Design review of the part built by this model. Coordinates are the model's own, in mm. A direction names the side the tool comes from. Give positions to 0.01 mm unless a question says otherwise; leave off trailing zeros. Write each loop counter-clockwise with the first axis right and the second up, starting at its lowest first coordinate (ties: lowest second). Pieces come first, ordered by that corner, then holes. Notation, with made-up numbers: (71, 3.25) -> (121, 3.25) arc R11 cw to (121, 19.25) -> close; hole circle Ø5 at (77.25, 57.5). An arc over 180 degrees is marked (long way). Write each question's results on one line, items separated by ' | '. Start each with the question number.
(1) Mouldability with a two-part tool opening along X and no side actions: class faces 1 (the face through (62.402, 13, 9)), 2 (the face through (-15.24, 1.65, 15.07)), 3 (the face through (23, 15, 20)) as released by +X, released by -X, zero draft, split by the parting line, or undercut.
(2) Take a section at C-C (z = 7.25). Count the separate pieces of the cut face and the enclosed holes in it, plus the area to 3 significant figures.
(3) Take a section at A-A (z = 12.75). State the section outline as (x, y) points.
(4) Take a section at B-B (y = 22). State the section outline as (x, z) points, plus the area to 3 significant figures.
(5) Clearance check with flat-ended pins moving along their axes: pin 1 (1.2 mm diameter, centred on y = 1.5, z = 4.5, fed in from -X); pin 2 (1.2 mm diameter, centred on x = 42, z = 6.5, fed in from -Y); pin 3 (1.2 mm diameter, centred on x = 12.5, y = 3, fed in from -Z). State where each tip first meets the part, or that it passes through.
(6) For faces 4 (the face through (57.165, 16.022, 5.07)), 5 (the face through (62.4, 31.32, 8.38)), 6 (the face through (16, 2, 10)), list the 3-axis set-ups (+Z, -Z, +X, -X, +Y, -Y) from which the entire face can be reached by the end or side of a thin tool; tool diameter is ignored.
(7) To check wall thickness, follow probe 1 along Y at (x, z) = (58.9, 5.25); probe 2 along Y at (x, z) = (42.4, 2.25); probe 3 along X at (y, z) = (8, 4.75). State the ranges of each line that lie inside material, in increasing order.
Autodesk Inventor part; units mm, degrees
ref_plane "YZ Plane" through (0, 0, 0) normal (1, 0, 0) x (0, 1, 0)
ref_plane "XZ Plane" through (0, 0, 0) normal (0, 1, 0) x (-1, 0, 0)
ref_plane "XY Plane" through (0, 0, 0) normal (0, 0, 1) x (1, 0, 0)
ref_plane "Arbeitsebene1" through (0, 0, 0) normal (0, 0, 1) x (1, 0, 0)
sketch "Skizze1" plane through (0, 0, 0) normal (0, 0, 1) x (1, 0, 0)
  line L0 (37.9, 26.5) -> (37.9, 13.35)
  line L1 (37.9, 13.35) -> (53.9, 13.35)
  line L2 (53.9, 13.35) -> (53.9, 13.85)
  line L3 (53.9, 13.85) -> (63.9, 13.85)
  line L4 (63.9, 13.85) -> (63.9, 27.75)
  arc A0 (63.9, 27.75) -> (58.9, 32.75) centre (58.9, 27.75) ccw
  line L5 (58.9, 32.75) -> (-58.9, 32.75)
  arc A1 (-58.9, 32.75) -> (-63.9, 27.75) centre (-58.9, 27.75) ccw
  line L6 (-63.9, 27.75) -> (-63.9, 19.25)
  line L7 (-63.9, 19.25) -> (-58.9, 19.25)
  line L8 (-58.9, 19.25) -> (-58.9, 19.75)
  line L9 (-58.9, 19.75) -> (-38.9, 19.75)
  line L10 (-38.9, 19.75) -> (-38.9, 13.85)
  line L11 (-38.9, 13.85) -> (-28.9, 13.85)
  line L12 (-28.9, 13.85) -> (-28.9, 13.35)
  line L13 (-28.9, 13.35) -> (-8.6, 13.35)
  line L14 (-8.6, 13.35) -> (-8.6, 26.5)
  line L15 (-8.6, 26.5) -> (37.9, 26.5)
  circle A2 centre (58.6204, 27.75) radius 1.4
  circle A3 centre (-59.1796, 27.75) radius 1.4
  circle A4 centre (-13.6, 16.25) radius 1.4
  circle A5 centre (-33.6, 16.25) radius 1.4
  circle A6 centre (58.9, 16.25) radius 1.4
  circle A7 centre (42.4, 16.25) radius 1.4
  line L16 (-8.6, -11.9682) -> (-10.6, -13.9682)
  line L17 (-8.6, -11.9682) -> (-8.6, 5.15)
  line L18 (-8.6, 5.15) -> (-28.9, 5.15)
  line L19 (-28.9, 5.15) -> (-28.9, 4.65)
  line L20 (-28.9, 4.65) -> (-38.9, 4.65)
  line L21 (-38.9, 4.65) -> (-38.9, -1.25)
  line L22 (-38.9, -1.25) -> (-58.9, -1.25)
  line L23 (-58.9, -1.25) -> (-58.9, -0.75)
  line L24 (-58.9, -0.75) -> (-63.9, -0.75)
  line L25 (-63.9, -0.75) -> (-63.9, -16.5797)
  arc A8 (-49.9, -11.2196) -> (-63.9, -16.5797) centre (-50.2702, -31.2162) ccw
  line L26 (-49.9, -11.2196) -> (-49.9, -13.9682)
  line L27 (-49.9, -13.9682) -> (-10.6, -13.9682)
  circle A9 centre (-13.3796, -11.2637) radius 1.4
  circle A10 centre (-33.6, 2.25) radius 1.4
  circle A11 centre (-13.6, 2.25) radius 1.4
  circle A12 centre (58.6204, -47.75) radius 1.4
  circle A13 centre (58.9, 2.25) radius 1.4
  circle A14 centre (42.4, 2.25) radius 1.4
  circle A15 centre (42.4, -11.2637) radius 1.4
  circle A16 centre (42.4, -31.25) radius 1.4
  line L28 (63.9, 4.65) -> (53.9, 4.65)
  line L29 (53.9, 4.65) -> (53.9, 5.15)
  line L30 (53.9, 5.15) -> (37.9, 5.15)
  line L31 (37.9, 5.15) -> (37.9, -41.35)
  line L32 (37.9, -41.35) -> (-33.0276, -41.35)
  arc A17 (-59.1255, -49.149) -> (-33.0276, -41.35) centre (-50.2702, -31.2162) ccw
  arc A18 (-60.3777, -48.4742) -> (-59.1255, -49.149) centre (-59.1796, -47.75) ccw
  arc A19 (-63.9, -45.8527) -> (-60.3777, -48.4742) centre (-50.2702, -31.2162) ccw
  line L33 (-63.9, -45.8527) -> (-63.9, -47.75)
  arc A20 (-63.9, -47.75) -> (-58.9, -52.75) centre (-58.9, -47.75) ccw
  line L34 (-58.9, -52.75) -> (58.9, -52.75)
  arc A21 (58.9, -52.75) -> (63.9, -47.75) centre (58.9, -47.75) ccw
  line L35 (63.9, -47.75) -> (63.9, 4.65)
  line L36 (-16.1, 32.75) -> (63.9, 32.75)
  line L37 (63.9, 32.75) -> (63.9, 0.75)
  line L38 (63.9, 0.75) -> (-16.1, 0.75)
  line L39 (-16.1, 0.75) -> (-16.1, 32.75)
  point P0 (0, 0)
  dimension "d0" = 80
  dimension "d1" = 0
  dimension "d2" = 32
extrude "Extrusion1" add sketch "Skizze1" along normal blind 20 contours L15 L14 L13 L39 L5 A0 L4 L3 L2 L1 L0 | L0 L1 L2 L3 L37 L28 L29 L30 L31 L38 L17 L18 L39 L13 L14 L15 | L18 L17 L38 L39 | L35 L38 L31 L30 L29 L28 | A2 | A4 | A6 | A7 | A11 | A13 | A14
fillet "Rundung1" radius 3 7 edges at (62.4355, 31.2855, 20) (63.9, 20.8, 20) (21.4, 32.75, 20) (-16.1, 16.75, 20) (-16.1, 0.75, 10) (-16.1, 32.75, 10) (63.9, 0.75, 10)
sketch "Skizze2" plane through (0, 0, 0) normal (0, 0, -1) x (-1, 0, 0)
  arc A0 (13.1, 0.75) -> (16.1, 3.75) centre (13.1, 3.75) ccw
  line L0 (16.1, 29.75) -> (16.1, 3.75)
  arc A1 (16.1, 29.75) -> (13.1, 32.75) centre (13.1, 29.75) ccw
  line L1 (-58.9, 32.75) -> (13.1, 32.75)
  arc A2 (-58.9, 32.75) -> (-63.9, 27.75) centre (-58.9, 27.75) ccw
  line L2 (-63.9, 3.75) -> (-63.9, 27.75)
  arc A3 (-63.9, 3.75) -> (-60.9, 0.75) centre (-60.9, 3.75) ccw
  line L3 (13.1, 0.75) -> (-60.9, 0.75)
  line L4 (63.9, -47.75) -> (63.9, 27.75)
  arc A4 (63.9, 27.75) -> (58.9, 32.75) centre (58.9, 27.75) ccw
  line L5 (58.9, 32.75) -> (-58.9, 32.75)
  arc A5 (-58.9, 32.75) -> (-63.9, 27.75) centre (-58.9, 27.75) ccw
  line L6 (-63.9, 27.75) -> (-63.9, -47.75)
  arc A6 (-63.9, -47.75) -> (-58.9, -52.75) centre (-58.9, -47.75) ccw
  line L7 (-58.9, -52.75) -> (58.9, -52.75)
  arc A7 (58.9, -52.75) -> (63.9, -47.75) centre (58.9, -47.75) ccw
  circle A8 centre (-42.4, -31.25) radius 1.4
  circle A9 centre (13.3796, -11.2637) radius 1.4
  circle A10 centre (-42.4, 16.25) radius 1.4
  circle A11 centre (-58.9, 16.25) radius 1.4
  circle A12 centre (-42.4, 2.25) radius 1.4
  circle A13 centre (33.6, 16.25) radius 1.4
  circle A14 centre (13.6, 2.25) radius 1.4
  circle A15 centre (13.6, 16.25) radius 1.4
  circle A16 centre (-58.9, 2.25) radius 1.4
  circle A17 centre (33.6, 2.25) radius 1.4
  circle A18 centre (-42.4, -11.2637) radius 1.4
  circle A19 centre (-58.6204, -47.75) radius 1.4
  circle A20 centre (59.1796, 27.75) radius 1.4
  circle A21 centre (59.1796, -47.75) radius 1.4
  circle A22 centre (-58.6204, 27.75) radius 1.4
  line L8 (-37.9, -41.35) -> (-37.9, 26.5)
  line L9 (-37.9, 26.5) -> (8.6, 26.5)
  line L10 (8.6, 26.5) -> (8.6, -11.9682)
  line L11 (10.6, -13.9682) -> (8.6, -11.9682)
  line L12 (10.6, -13.9682) -> (49.9, -13.9682)
  line L13 (49.9, -13.9682) -> (49.9, -41.35)
  line L14 (49.9, -41.35) -> (-37.9, -41.35)
  line L15 (58.9, -0.75) -> (58.9, -1.25)
  line L16 (58.9, -1.25) -> (38.9, -1.25)
  line L17 (38.9, -1.25) -> (38.9, 19.75)
  line L18 (38.9, 19.75) -> (58.9, 19.75)
  line L19 (58.9, 19.75) -> (58.9, 19.25)
  line L20 (58.9, 19.25) -> (55.9, 19.25)
  line L21 (55.9, -0.75) -> (55.9, 19.25)
  line L22 (58.9, -0.75) -> (55.9, -0.75)
  point P0 (0, 0)
hole "Bohrung1" at (42.4, 2.25, 0) at (58.9, 2.25, 0) at (58.9, 16.25, 0) at (42.4, 16.25, 0) at (58.6204, 27.75, 0) at (-13.6, 16.25, 0) at (-13.6, 2.25, 0) direction (0, 0, 1) diameter 3.5 depth 10 tip angle 118
sketch "Skizze3" plane through (0, 0, 0) normal (0, 0, -1) x (-1, 0, 0)
  arc A0 (15.2448, 1.6524) -> (16.1, 3.75) centre (13.1, 3.75) ccw
  line L0 (16.1, 29.75) -> (16.1, 3.75)
  arc A1 (16.1, 29.75) -> (13.1, 32.75) centre (13.1, 29.75) ccw
  line L1 (-58.9, 32.75) -> (13.1, 32.75)
  arc A2 (-58.9, 32.75) -> (-63.9, 27.75) centre (-58.9, 27.75) ccw
  line L2 (-63.9, 3.75) -> (-63.9, 27.75)
  arc A3 (-63.9, 3.75) -> (-60.9, 0.75) centre (-60.9, 3.75) ccw
  line L3 (-43.3014, 0.75) -> (-57.9986, 0.75)
  arc A4 (-58.9, 31.2519) -> (-62.4019, 27.75) centre (-58.9, 27.75) ccw
  line L4 (-58.9, 31.2519) -> (13.1, 31.2519)
  arc A5 (14.6019, 29.75) -> (13.1, 31.2519) centre (13.1, 29.75) ccw
  line L5 (14.6019, 29.75) -> (14.6019, 5.3398)
  arc A6 (14.6019, 5.3398) -> (10.3519, 2.2481) centre (13.6, 2.25) ccw
  line L6 (10.3519, 2.2481) -> (-39.1519, 2.2481)
  arc A7 (-39.1519, 2.2481) -> (-45.6481, 2.2481) centre (-42.4, 2.25) ccw
  line L7 (-45.6481, 2.2481) -> (-55.6519, 2.2481)
  arc A8 (-55.6519, 2.2481) -> (-62.0942, 2.8393) centre (-58.9, 2.25) ccw
  arc A9 (-62.4019, 3.75) -> (-62.0942, 2.8393) centre (-60.9, 3.75) ccw
  line L8 (-62.4019, 3.75) -> (-62.4019, 27.75)
  circle A10 centre (-58.9, 16.25) radius 3.4626
  circle A11 centre (-58.6204, 27.75) radius 3.6913
  circle A12 centre (-42.4, 16.25) radius 3.7166
  circle A13 centre (13.6, 16.25) radius 4.3613
  arc A14 (15.2448, 1.6524) -> (12.6986, 0.75) centre (13.6, 2.25) ccw
  line L9 (-59.8014, 0.75) -> (-60.9, 0.75)
  arc A15 (-57.9986, 0.75) -> (-59.8014, 0.75) centre (-58.9, 2.25) ccw
  arc A16 (-41.4986, 0.75) -> (-43.3014, 0.75) centre (-42.4, 2.25) ccw
  line L10 (12.6986, 0.75) -> (-41.4986, 0.75)
  point P0 (0, 0)
  point P1 (-57.4529, 31.2519)
  point P2 (-61.1978, 30.3926)
  point P3 (-61.7336, 4.9993)
  point P4 (14.6019, 12.0053)
  point P5 (14.6019, 20.4947)
extrude "Extrusion2" cut sketch "Skizze3" against normal blind 18 contours L5 A6 L6 A7 L7 A8 A9 L8 A4 A11 L4 A5 A13
sketch "Skizze4" plane through (-13.1, 0.75, 20) normal (0, -1, 0) x (1, 0, 0)
  circle A0 centre (31.7066, -26.8441) radius 6
  line L0 (45.2066, -35.8441) -> (18.2066, -35.8441)
  line L1 (18.2066, -35.8441) -> (18.2066, -17.8441)
  line L2 (18.2066, -17.8441) -> (45.2066, -17.8441)
  line L3 (45.2066, -17.8441) -> (45.2066, -35.8441)
  line L4 (45.2066, -35.8441) -> (18.2066, -17.8441) construction
  line L5 (18.2066, -35.8441) -> (45.2066, -17.8441) construction
  point P0 (13.1, -20)
  dimension "d15" = 27
  dimension "d16" = 18
extrude "Extrusion3" cut sketch "Skizze4" against normal blind 18 contours A0 | L0 L1 L2 L3
sketch "Sketch5" plane through (-13.1, 0.75, 20) normal (0, -1, 0) x (1, 0, 0)
  line L0 (-5, -20) -> (61, -20)
  line L1 (61, -20) -> (61, -10)
  line L2 (61, -10) -> (-5, -10)
  line L3 (-5, -10) -> (-5, -20)
  point P0 (13.1, -20)
extrude "Extrusion4" cut sketch "Sketch5" against normal blind 4
properties part number "10_Wellplate_base_Lasercover"
Report:
1) face 1: undercut | face 2: released by -X | face 3: zero draft
2) separate pieces: 4 | enclosed holes: 4 | area: 356 mm2
3) outline: (-16.1, 3.75) arc R3 ccw to (-13.1, 0.75) -> (60.9, 0.75) arc R3 ccw to (63.9, 3.75) -> (63.9, 27.75) arc R5 ccw to (58.9, 32.75) -> (-13.1, 32.75) arc R3 ccw to (-16.1, 29.75) -> close; circle Ø7.43 at (42.4, 16.25); circle Ø6.93 at (58.9, 16.25); hole (-14.6, 5.34) arc R3.25 cw to (-10.35, 2.25) -> (39.15, 2.25) arc R3.25 cw to (45.65, 2.25) -> (55.65, 2.25) arc R3.25 cw to (62.09, 2.84) arc R1.5 ccw to (62.4, 3.75) -> (62.4, 27.75) arc R3.5 ccw to (61.2, 30.39) arc R3.69 cw (long way) to (57.45, 31.25) -> (-13.1, 31.25) arc R1.5 ccw to (-14.6, 29.75) -> (-14.6, 20.49) arc R4.36 cw (long way) to (-14.6, 12.01) -> close
4) outline: (-16.1, 0) -> (-14.6, 0) -> (-14.6, 18) -> (62.4, 18) -> (62.4, 0) -> (63.9, 0) -> (63.9, 17) arc R3 ccw to (60.9, 20) -> (-13.1, 20) arc R3 ccw to (-16.1, 17) -> close | area: 210 mm2
5) pin 1: x = 47.9 | pin 2: y = 4.75 | pin 3: z = 18
6) face 4: -Z | face 5: +Z, -Z, +X, +Y | face 6: -Z, -X, -Y
7) probe 1: 4 to 5.5, 12.79 to 14.5, 18 to 19.71, 24.07 to 26.02, 29.48 to 32.75 | probe 2: 4.75 to 5.5, 12.53 to 14.5, 18 to 19.97, 31.25 to 32.75 | probe 3: -16.1 to -14.6, 62.4 to 63.9
